from build123d import *

# Parameters (mm, degrees)
BOSS_EXTRUDE1_DEPTH = 5.2
BOSS_EXTRUDE2_DEPTH = 5.2
BOSS_EXTRUDE3_DEPTH = 12.7


with BuildPart() as part:
    # Sketch1 → Boss-Extrude1 (new body)
    with BuildSketch(Plane(origin=(0, 0, 0), x_dir=(1, 0, 0), z_dir=(0, 1, 0))):
        with BuildLine():
            Line((0, 2.29), (0, -2.29))
            ThreePointArc((0, -2.29), (-2.29, 0), (0, 2.29))
        make_face()
    extrude(amount=BOSS_EXTRUDE1_DEPTH)

    # Sketch1_3 → Boss-Extrude2 (add)
    with BuildSketch(Plane(origin=(0, 0, 0), x_dir=(1, 0, 0), z_dir=(0, 1, 0))):
        Polygon((1.4, 2.044905497), (1.4, -2.044905497), (0.01, -2.29), (0, -2.29), (0, 2.29), (0.01, 2.29), align=None)
    extrude(amount=BOSS_EXTRUDE2_DEPTH)

    # Sketch3 → Boss-Extrude3 (add)
    with BuildSketch(Plane.XZ):
        Polygon((0, -1.02), (0, -1.52), (-0.5, -1.52), (-0.5, -1.27), (-0.5, -1.02), align=None)
        Polygon((0, 0.25), (0, -0.25), (-0.5, -0.25), (-0.5, 0), (-0.5, 0.25), align=None)
        Polygon((0, 1.52), (0, 1.02), (-0.5, 1.02), (-0.5, 1.27), (-0.5, 1.52), align=None)
    extrude(amount=BOSS_EXTRUDE3_DEPTH)


solid = part.part
Here's how the part is built. I have some questions about the finished solid (model axes, mm). Give positions to 0.01 mm unless a question says otherwise; leave off trailing zeros. Order: outer loops, then holes, each group sorted by start corner. A loop starts at its lowest first (then second) coordinate and runs counter-clockwise, first axis right, second up. Notation, with made-up numbers: M -28.5,23 L -9.5,23 A23 cw -9.5,43 Z; hole C -40,-27.5 d6. An arc over 180 degrees is marked long. Answer as a JSON object with one key per item and string values. Group by question number.
1) Suppose I cut it at B-B, the plane z = 0. Write out the boundary of the cut face in (x, y), plus the area to 3 significant figures.
2) Suppose I cut it at D-D, the plane x = -0.25. Write out the boundary of the cut face in (y, z).
3) Suppose I cut it at A-A, the plane y = -0.75. Write out the boundary of the cut face in (x, z), plus the area to 3 significant figures.
4) I'm going to push flat-ended pins straight in: pin 1 Ø1.5 at (x, y) = (0.5, -3) entering from -Z; pin 2 Ø0.6 at (y, z) = (-4, -1) entering from -X; pin 3 Ø0.6 at (x, y) = (-0.5, -7) entering from +Z. Where does each tip first touch, or does it pass through?
5) Please list where these lines run through material, in increasing order: L1, parallel to Z at x = -0.2, y = -7.25; L2, parallel to Y at x = -0.9, z = 1.3; L3, parallel to X at y = -10.75, z = 0. Write a range as [from, to].
Results found:
{
 "1": {"outline": "M -2.29,0 L -0.5,0 L -0.5,-12.7 L 0,-12.7 L 0,0 L 1.4,0 L 1.4,5.2 L -2.29,5.2 Z", "area": "25.5 mm²"},
 "2": {"outline": "M -12.7,-1.52 L 0,-1.52 L 0,-2.28 L 5.2,-2.28 L 5.2,2.28 L 0,2.28 L 0,1.52 L -12.7,1.52 L -12.7,1.02 L 0,1.02 L 0,0.25 L -12.7,0.25 L -12.7,-0.25 L 0,-0.25 L 0,-1.02 L -12.7,-1.02 Z"},
 "3": {"outline": "M -0.5,-1.52 L 0,-1.52 L 0,-1.02 L -0.5,-1.02 Z; M -0.5,-0.25 L 0,-0.25 L 0,0.25 L -0.5,0.25 Z; M -0.5,1.02 L 0,1.02 L 0,1.52 L -0.5,1.52 Z", "area": "0.750 mm²"},
 "4": {"pin 1": "z = -1.52", "pin 2": "x = -0.5", "pin 3": "z = 1.52"},
 "5": {"L1": "[-1.52, -1.02], [-0.25, 0.25], [1.02, 1.52]", "L2": "[0, 5.2]", "L3": "[-0.5, 0]"}
}
